from build123d import *

# Parameters (mm, degrees)
IZIM1_R                          = 2
Y_KSEKLIK_EKSTR_ZYON1_DEPTH      = 4
IZIM1_3_R                        = 0.75
Y_KSEKLIK_EKSTR_ZYON2_DEPTH      = 4
Y_KSEKLIK_EKSTR_ZYON2_DEPTH_BACK = 68


with BuildPart() as part:
    # izim1 → Y_kseklik-Ekstr_zyon1 (new body)
    with BuildSketch(Plane.XY):
        with BuildLine():
            Line((-0.74712339, 20.065625), (-2.490411299, 0.21875))
            ThreePointArc((-2.490411299, 0.21875), (0, -2.5), (2.490411299, 0.21875))
            Line((2.490411299, 0.21875), (0.74712339, 20.065625))
            ThreePointArc((0.74712339, 20.065625), (0, 19.25), (-0.74712339, 20.065625))
        make_face()
        Circle(IZIM1_R, mode=Mode.SUBTRACT)
    extrude(amount=Y_KSEKLIK_EKSTR_ZYON1_DEPTH)

    # izim1_3 → Y_kseklik-Ekstr_zyon2 (add, two sides)
    with BuildSketch(Plane.XY) as y_kseklik_ekstr_zyon2_sk:
        with Locations((0, 20)):
            Circle(IZIM1_3_R)
    extrude(amount=Y_KSEKLIK_EKSTR_ZYON2_DEPTH)
    extrude(y_kseklik_ekstr_zyon2_sk.sketch, amount=-Y_KSEKLIK_EKSTR_ZYON2_DEPTH_BACK)


solid = part.part
Read the model definition and answer for the solid it produces. Units are mm, in the model's axes. A direction names the side the tool comes from. Round coordinates to 2 decimals unless told otherwise and drop trailing zeros. Write each loop counter-clockwise with the first axis right and the second up, starting at its lowest first coordinate (ties: lowest second). Pieces come first, ordered by that corner, then holes. Notation, with made-up numbers: (17.5, 28.5) - (64.5, 28.5) arc R18 ccw to (64.5, 52.5) - close; hole circle Ø7 at (31, 82.25). An arc over 180 degrees is marked (long way). One line per question, with ' | ' between items. Start each with the question number.
1. Section C-C (y = 17) is taken. Determine the outline of the cut face in (x, z), and give its area (3 significant figures).
2. Each of these flat-tipped pins is pushed along its axis until it touches: pin 1 (6 mm diameter, centred on y = 18.5, z = -35.5, fed in from -X); pin 2 (1.5 mm diameter, centred on x = 0, y = 14.5, fed in from -Z). Where does it stop, or does it pass through?
3. For faces 1 (the face through (0.403, 20.632, -31.496)), 2 (the face through (1.63, 10, 1.97)), determine the directions among +Z, -Z, +X, -X, +Y, -Y from which every point of the face is accessible in a straight line to the end or side of a thin tool.
4. Find the intervals of material crossed by probe 1 along Y at (x, z) = (0, 1.1); probe 2 along Z at (x, y) = (1.3, 12.25); probe 3 along X at (y, z) = (19.5, -50.5), in increasing order. Write a range as [from, to].
5. Section A-A (x = 0) is taken. Determine the outline of the cut face in (y, z).
6. Section B-B (z = -18) is taken. Determine the outline of the cut face in (x, y), and give its area (3 significant figures).
7. For a pull along X with two mould halves and no side action, classify faces 3 (the face through (0, 9, 4)), 4 (the face through (0, -2, 2)), 5 (the face through (-1.607, 10.281, 1.972)) as +X half, -X half, draft (parallel to the pull), parting line (faces both ways), or undercut.
Filled in:
1) outline: (-1.02, 0) - (1.02, 0) - (1.02, 4) - (-1.02, 4) - close | area: 8.13 mm²
2) pin 1: x = -0.75 | pin 2: z = 0
3) face 1: -Z | face 2: +Z, -Z, +X, +Y
4) probe 1: [-2.5, -2], [2, 20.75] | probe 2: [0, 4] | probe 3: [-0.56, 0.56]
5) outline: (-2.5, 0) - (-2, 0) - (-2, 4) - (-2.5, 4) - close; (2, 0) - (19.25, 0) - (19.25, -68) - (20.75, -68) - (20.75, 4) - (2, 4) - close
6) outline: circle Ø1.5 at (0, 20) | area: 1.77 mm²
7) face 3: draft | face 4: undercut | face 5: -X half
